Here's how the part is built. I have some questions about the finished solid (model axes, mm). Round coordinates to 2 decimals unless told otherwise and drop trailing zeros. Write each loop counter-clockwise with the first axis right and the second up, starting at its lowest first coordinate (ties: lowest second). Pieces come first, ordered by that corner, then holes. Notation, with made-up numbers: (75, -0.5) -> (104, -0.5) arc R21 cw to (104, 19.5) -> close; hole circle Ø6 at (4, 76.25). An arc over 180 degrees is marked (long way). Put each result on its own line as item: value. Start each with the question number.
1) If I drill on line 1 along X through (y, z) = (31, 1.9); line 2 along X through (y, z) = (61.5, 1.6); line 3 along X through (y, z) = (29, 1.6), over which ranges is the centre line in solid material (lowest first)? Write a range as [from, to].
2) I want a section at C-C, the plane x = 0. List the corners of the cut face in (y, z) for me, then the cut area to 3 significant figures.
3) I want a section at B-B, the plane z = 0.6. List the corners of the cut face in (x, y) for me, then the cut area to 3 significant figures.
4) I want a section at D-D, the plane y = 57. List the corners of the cut face in (x, z) for me.
5) I want a section at A-A, the plane y = 35.5. List the corners of the cut face in (x, z) for me, then the cut area to 3 significant figures.
6) Will these pins go through, and if not, where does the flat tip stop? P1, Ø1.5, axis at y = 11, z = 3, coming from the +X side; P2, Ø1, axis at y = 46.5, z = 1, coming from the +X side; P3, Ø2.5, axis at x = -44.19, y = 44.19, coming from the -Z side.
Autodesk Inventor part; units mm, degrees
ref_plane "YZ Plane" through (0, 0, 0) normal (1, 0, 0) x (0, 1, 0)
ref_plane "XZ Plane" through (0, 0, 0) normal (0, 1, 0) x (-1, 0, 0)
ref_plane "XY Plane" through (0, 0, 0) normal (0, 0, 1) x (1, 0, 0)
sketch "スケッチ5" plane through (0, 0, 3.2) normal (0, 0, 1) x (1, 0, 0)
  circle A0 centre (-16.1762, 60.3704) radius 1.621
  circle A1 centre (16.1762, 60.3704) radius 1.621
  arc A2 (67.5, 0) -> (-67.5, 0) centre (0, 0) ccw
  circle A3 centre (-16.1762, 60.3704) radius 5
  circle A4 centre (16.1762, 60.3704) radius 5
  circle A5 centre (-44.1942, 44.1942) radius 1.621
  circle A6 centre (-60.3704, 16.1762) radius 1.621
  circle A7 centre (44.1942, 44.1942) radius 1.621
  circle A8 centre (60.3704, 16.1762) radius 1.621
  arc A9 (62.5, 0) -> (-62.5, 0) centre (0, 0) ccw
  circle A10 centre (-44.1942, 44.1942) radius 5
  circle A11 centre (-60.3704, 16.1762) radius 5
  circle A12 centre (44.1942, 44.1942) radius 5
  circle A13 centre (60.3704, 16.1762) radius 5
  line L0 (-45.5, 0) -> (-67.5, 0)
  line L1 (67.5, 0) -> (45.5, 0)
  point P0 (17.4703, 65.2)
  point P1 (-17.4703, 65.2)
  point P2 (58.8841, 20.9502)
  point P3 (65.2, 17.4703)
  point P4 (47.7297, 47.7297)
  point P5 (47.5855, 40.52)
  point P6 (40.52, 47.5855)
  point P7 (20.9502, 58.8841)
  point P8 (-65.2, 17.4703)
  point P9 (-58.8841, 20.9502)
  point P10 (-47.5855, 40.52)
  point P11 (-47.7297, 47.7297)
  point P12 (-40.52, 47.5855)
  point P13 (-20.9502, 58.8841)
  point P14 (-11.2987, 61.4702)
  point P15 (11.2987, 61.4702)
  point P16 (61.4702, 11.2987)
  point P17 (-61.4702, 11.2987)
sketch "スケッチ1" plane through (0, 0, 0) normal (0, 0, 1) x (1, 0, 0)
  arc A0 (45.456, 2) -> (-45.5, 0) centre (0, 0) ccw
  arc A1 (67.5, 0) -> (-67.5, 0) centre (0, 0) ccw
  arc A2 (67.4704, -2) -> (-67.4704, -2) centre (0, 0) ccw
  arc A3 (45.456, 2) -> (-45.456, 2) centre (0, 0) ccw
  line L0 (-56.5, 2) -> (-56.5, -2)
  line L1 (-56.5, 2) -> (-45.456, 2)
  line L2 (-56.5, -2) -> (-67.4704, -2)
  line L3 (0, 81.4) -> (0, -15.9)
  line L4 (56.5, 2) -> (56.5, -2)
  line L5 (56.5, 2) -> (45.456, 2)
  line L6 (56.5, -2) -> (67.4704, -2)
  line L7 (-45.5, 0) -> (0, 0)
  point P0 (44.5, 0)
  point P1 (45.5, 0)
  dimension "d0" = 91
  dimension "d1" = 135
  dimension "d58" = 11
  dimension "d61" = 2
  dimension "d62" = 2
extrude "プレート2" add sketch "スケッチ1" along normal blind 3.2 contours L1 L0 L2 A2 A1 L3 A0 | L3 A1 A2 L6 L4 L5 A0
sketch "スケッチ2" plane through (0, 0, 3.2) normal (0, 0, 1) x (1, 0, 0)
  circle A0 centre (0, 0) radius 62.5
  point P0 (16.1762, 60.3704)
  point P1 (-16.1762, 60.3704)
  point P2 (-44.1942, 44.1942)
  point P3 (-60.3704, 16.1762)
  point P4 (-60.3704, -16.1762)
  point P5 (-44.1942, -44.1942)
  point P6 (-16.1762, -60.3704)
  point P7 (16.1762, -60.3704)
  point P8 (44.1942, -44.1942)
  point P9 (60.3704, -16.1762)
  point P10 (60.3704, 16.1762)
  point P11 (44.1942, 44.1942)
  dimension "d8" = 125
  dimension "d11" = 360
  dimension "d49" = 0
hole "穴1" at (16.1762, 60.3704, 3.2) at (-16.1762, 60.3704, 3.2) at (-44.1942, 44.1942, 3.2) at (-60.3704, 16.1762, 3.2) at (-60.3704, -16.1762, 3.2) at (-44.1942, -44.1942, 3.2) at (-16.1762, -60.3704, 3.2) at (16.1762, -60.3704, 3.2) at (44.1942, -44.1942, 3.2) at (60.3704, -16.1762, 3.2) at (60.3704, 16.1762, 3.2) at (44.1942, 44.1942, 3.2) direction (0, 0, -1) diameter 3.242 end through all
sketch "スケッチ6" plane through (0, 0, 3.2) normal (0, 0, 1) x (1, 0, 0)
  line L0 (-32.1734, 32.1734) -> (-29.3449, 29.3449)
  line L1 (29.3449, 29.3449) -> (32.1734, 32.1734)
  line L2 (0, 81.4) -> (0, -15.9)
  arc A0 (29.3449, 29.3449) -> (-29.3449, 29.3449) centre (0, 0) ccw
  arc A1 (45.456, 2) -> (-45.456, 2) centre (0, 0) ccw
  line L3 (-29.3449, 29.3449) -> (0, 0) construction
  line L4 (0, 0) -> (29.3449, 29.3449) construction
  point P0 (29.3449, 29.3449)
  dimension "d50" = 45
  dimension "d51" = 45
  dimension "d64" = 4
extrude "押し出し2" add sketch "スケッチ6" against normal up to surface (3.2 mm away)
fillet "コーナーR7" radius 1 4 edges at (-32.1734, 32.1734, 1.6) (-29.3449, 29.3449, 1.6) (32.1734, 32.1734, 1.6) (29.3449, 29.3449, 1.6)
fillet "コーナーR8" radius 1 4 edges at (-56.5, 2, 1.6) (56.5, 2, 1.6) (-56.5, -2, 1.6) (56.5, -2, 1.6)
equation "\"d18\" = Thickness"
equation "\"d6\" = Thickness"
equation "\"BendRadius\" = Thickness"
equation "\"BendReliefWidth\" = Thickness"
equation "\"BendReliefDepth\" = 0.5 * Thickness"
equation "\"CornerReliefSize\" = 4 * Thickness"
equation "\"MinimumRemnant\" = 2 * Thickness"
equation "\"TransitionRadius\" = BendRadius"
equation "\"JacobiRadiusSize\" = BendRadius"
equation "\"GapSize\" = Thickness"
properties part number "plate1" material "鋼、炭素鋼"
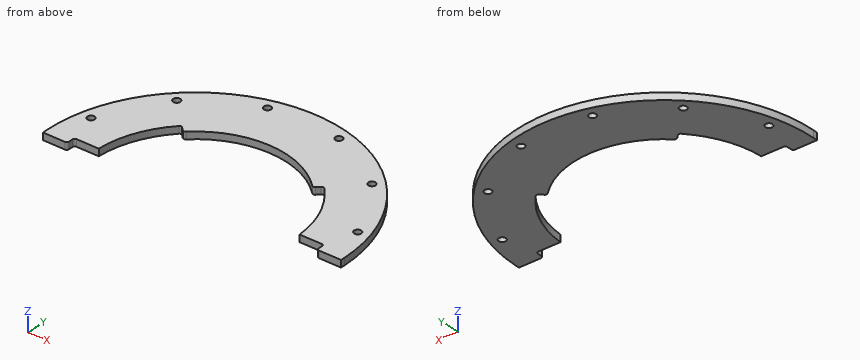
Findings:
1. line 1: x = [-59.96, -33.31], [-31, -27.59], [27.59, 31], [33.31, 59.96]
1. line 2: x = [-27.82, -17.34], [-15.01, 15.01], [17.34, 27.82]
1. line 3: x = [-60.95, -35.06], [35.06, 60.95]
2. outline: (41.5, 0) -> (67.5, 0) -> (67.5, 3.2) -> (41.5, 3.2) -> close
2. area: 83.2 mm2
3. outline: (-67.47, -2) -> (-57.5, -2) arc R1 ccw to (-56.5, -1) -> (-56.5, 1) arc R1 cw to (-55.5, 2) -> (-45.46, 2) arc R45.5 cw to (-32.89, 31.44) arc R1 cw to (-31.46, 31.46) -> (-30.04, 30.04) arc R1 ccw to (-28.65, 30.03) arc R41.5 cw to (28.65, 30.03) arc R1 ccw to (30.04, 30.04) -> (31.46, 31.46) arc R1 cw to (32.89, 31.44) arc R45.5 cw to (45.46, 2) -> (55.5, 2) arc R1 cw to (56.5, 1) -> (56.5, -1) arc R1 ccw to (57.5, -2) -> (67.47, -2) arc R67.5 ccw (long way) to start; hole circle Ø3.24 at (-60.37, 16.18); hole circle Ø3.24 at (-44.19, 44.19); hole circle Ø3.24 at (-16.18, 60.37); hole circle Ø3.24 at (16.18, 60.37); hole circle Ø3.24 at (44.19, 44.19); hole circle Ø3.24 at (60.37, 16.18)
3. area: 4,130 mm2
4. outline: (-36.16, 0) -> (36.16, 0) -> (36.16, 3.2) -> (-36.16, 3.2) -> close
5. outline: (-57.41, 0) -> (-21.49, 0) -> (-21.49, 3.2) -> (-57.41, 3.2) -> close; (21.49, 0) -> (57.41, 0) -> (57.41, 3.2) -> (21.49, 3.2) -> close
5. area: 230 mm2
6. P1: stops at x = 66.72
6. P2: stops at x = 49.4
6. P3: passes through
